The model under review builds one solid part; all positions refer to its coordinate system, in mm. A direction names the side the tool comes from. Coordinates: 2 decimals unless noted, no trailing zeros. Loops run counter-clockwise (first coordinate to the right, second up) from the corner with the lowest first, then second, coordinate; pieces in that order, holes last. Notation, with made-up numbers: M 43,57 L 55,57 A9 cw 55,67 Z; hole C 33.5,10 d2. An arc over 180 degrees is marked long. Return JSON: item names as keys, results as strings.
Autodesk Inventor part; units mm, degrees
ref_plane "YZ Plane" through (0, 0, 0) normal (1, 0, 0) x (0, 1, 0)
ref_plane "XZ Plane" through (0, 0, 0) normal (0, 1, 0) x (-1, 0, 0)
ref_plane "XY Plane" through (0, 0, 0) normal (0, 0, 1) x (1, 0, 0)
sketch "Sketch1" plane through (0, 0, 0) normal (0, 1, 0) x (-1, 0, 0)
  line L0 (0, 0) -> (-9.3015, 0)
  line L1 (7.5, -14) -> (0, -14)
  line L2 (13, -19) -> (13, -16)
  line L3 (7.5, -16) -> (7.5, -14)
  line L4 (13, -19) -> (3, -19)
  line L5 (3, -19) -> (3, -17.4)
  line L6 (3, -17.4) -> (1, -17.4)
  line L7 (1, -17.4) -> (1, -19)
  line L8 (-22.5, -51.5) -> (-27.5, -51.5)
  line L9 (-27.5, -51.5) -> (-27.5, -41.5)
  line L10 (-27.5, -41.5) -> (0, -14)
  line L11 (13, -16) -> (11.5, -16)
  line L12 (11.5, -16) -> (11.5, -17)
  line L13 (11.5, -17) -> (10.5, -17)
  line L14 (10.5, -17) -> (10.5, -16)
  line L15 (10.5, -16) -> (7.5, -16)
  line L16 (-22.5, -51.5) -> (-22.5, -42.5)
  line L17 (-22.5, -42.5) -> (1, -19)
  point P0 (25, -13.6173)
  dimension "d2" = 28
  dimension "d19" = 103
  dimension "d20" = 83
  dimension "d21" = 5
  dimension "d22" = 1.6
  dimension "d23" = 135
  dimension "d24" = 2
  dimension "d25" = 1
  dimension "d26" = 1
  dimension "d27" = 3
  dimension "d28" = 1.5
  dimension "d29" = 38
  dimension "d30" = 2
  dimension "d32" = 10
  dimension "d33" = 9
revolve "Revolution1" add sketch "Sketch1" angle 360 about axis through (0, 0, 0) along (1, 0, 0)
thread "Thread4"
sketch "Sketch2" plane through (22.5, 0, 0) normal (-1, 0, 0) x (0, 0, 1)
  point P0 (0, 0)
  point P1 (48, 0)
  dimension "d36" = 48
hole "Hole1" at (22.5, 0, 48) direction (1, 0, 0) diameter 3.5 depth 5
pattern_circular "Circular Pattern1" count 6 over 360 about axis through (25, 0, 0) along (1, 0, 0) of "Hole1"
properties part number "027" material "Aluminum 6061"
1. Add section B-B on y = 0. State how many separate pieces and enclosed holes the cut face has, plus the area to 3 significant figures.
Check values:
{"separate pieces": "4", "enclosed holes": "0", "area": "461 mm²"}
2. The part is to be moulded in two halves that separate along Z. For faces 1 (the face through (25.035, 0.67, 49.617)), 2 (the face through (-1, -17, -6)), 3 (the face through (25.035, -50.275, 11.164)), say which applies: released by +Z, released by -Z, zero draft, split by the parting line, or undercut.
Check values:
{"face 1": "undercut", "face 2": "zero draft", "face 3": "split by the parting line"}
3. To check wall thickness, follow line 1 (Y direction, x = 26, z = 24); line 2 (Y direction, x = 26.25, z = 24); line 3 (X direction, y = -8.5, z = 47). State the ranges of each line that lie inside material, in increasing order.
Check values:
{"line 1": "-45.57 to -43.32, -39.82 to -32, 32 to 39.82, 43.32 to 45.57", "line 2": "-45.57 to -43.32, -39.82 to -32.31, 32.31 to 39.82, 43.32 to 45.57", "line 3": "22.5 to 27.5"}
4. Machinability: for faces 4 (the face through (-10.5, -10, -13)), 5 (the face through (25.04, 42.63, -25.39)), 6 (the face through (22.5, -18.8, 38.4)), which of the approach directions +Z, -Z, +X, -X, +Y, -Y give a long, thin tool a straight path to every point of the face, cutting with its end or side? Answer none if there is none.
Check values:
{"face 4": "none", "face 5": "+X, -X", "face 6": "-X"}
5. Add section D-D on z = 48. Give the boundary of the cut face in (x, y), plus the area to 3 significant figures.
Check values:
{"outline": "M 22.5,-18.66 L 27.5,-18.66 L 27.5,-1.75 L 22.5,-1.75 Z; M 22.5,1.75 L 27.5,1.75 L 27.5,18.66 L 22.5,18.66 Z", "area": "169 mm²"}
6. Insertion check: pin 1 Ø4.5 at (y, z) = (41.57, -24) entering from -X; pin 2 Ø1.5 at (x, y) = (18.5, -33) entering from -Z; pin 3 Ø10 at (x, z) = (16, 9) entering from -Y. Each pin has a flat end and moves straight along its axis. Give the tip position at first contact, or say it passes through.
Check values:
{"pin 1": "x = 22.5", "pin 2": "z = -21.67", "pin 3": "y = -40.11"}
7. Add section C-C on x = -5. Give the boundary of the cut face in (y, z).
Check values:
{"outline": "C 0,0 d38; hole C 0,0 d28"}
